Can you work these out from the drawing? Everything is in mm from the part's minimum corner. A direction names the side the tool comes from. Round coordinates to 2 decimals unless told otherwise and drop trailing zeros. Loops run counter-clockwise (first coordinate to the right, second up) from the corner with the lowest first, then second, coordinate; pieces in that order, holes last. Notation, with made-up numbers: M 48,5.25 L 55,5.25 A15 ccw 55,12.25 Z; hole C 0,60.25 d7. An arc over 180 degrees is marked long. Use a Markdown table: item, result.
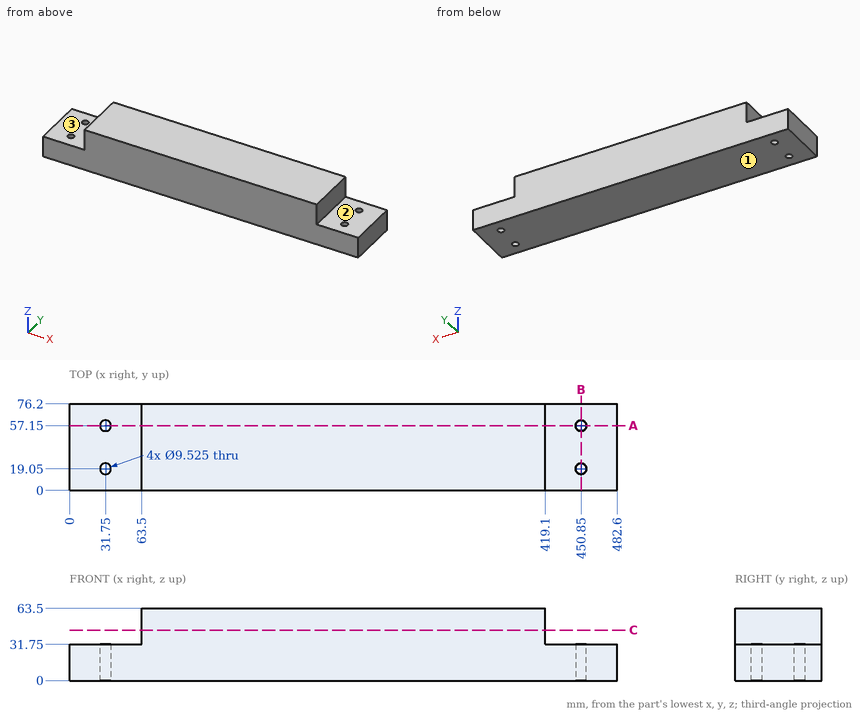
1. Which directions (+Z, -Z, +X, -X, +Y, -Y) give clear straight access to the entire face, cutting with the end or side of a thin tool? Please do the marked faces 1, 2 and 3.
Answer sheet:
| item | result |
|---|---|
| face 1 | -Z, +X, -X, +Y, -Y |
| face 2 | +Z, +X, +Y, -Y |
| face 3 | +Z, -X, +Y, -Y |
2. For pin 1 Ø16 at (y, z) = (40, 50) entering from +X; pin 2 Ø8.5 at (x, y) = (450.85, 57.15) entering from +Z; pin 3 Ø12 at (y, z) = (38.5, 45) entering from -X; pin 4 Ø19 at (x, y) = (20, 39) entering from +Z, each with a flat end and sliding along its axis, tell me the tip position at first contact or that it passes through.
Answer sheet:
| item | result |
|---|---|
| pin 1 | x = 419.1 |
| pin 2 | through |
| pin 3 | x = 63.5 |
| pin 4 | z = 31.75 |
3. Imagine slicing it at C-C, the plane z = 44.5. Write out the boundary of the cut face in (x, y), then the cut area to 3 significant figures.
Answer sheet:
| item | result |
|---|---|
| outline | M 63.5,0 L 419.1,0 L 419.1,76.2 L 63.5,76.2 Z |
| area | 27,100 mm2 |
4. Imagine slicing it at B-B, the plane x = 450.85. Write out the boundary of the cut face in (y, z).
Answer sheet:
| item | result |
|---|---|
| outline | M 0,0 L 14.29,0 L 14.29,31.75 L 0,31.75 Z; M 23.81,0 L 52.39,0 L 52.39,31.75 L 23.81,31.75 Z; M 61.91,0 L 76.2,0 L 76.2,31.75 L 61.91,31.75 Z |
5. I need wall thicknesses on probe 1 along Y at (x, z) = (31.75, 21); probe 2 along X at (y, z) = (19, 23); probe 3 along X at (y, z) = (15, 15). Which ranges of each line are inside material? Lowest first, please. Write a range as from..to.
Answer sheet:
| item | result |
|---|---|
| probe 1 | 0..14.29, 23.81..52.39, 61.91..76.2 |
| probe 2 | 0..26.99, 36.51..446.09, 455.61..482.6 |
| probe 3 | 0..29.24, 34.26..448.34, 453.36..482.6 |
6. Imagine slicing it at A-A, the plane y = 57.15. Write out the boundary of the cut face in (x, z), then the cut area to 3 significant figures.
Answer sheet:
| item | result |
|---|---|
| outline | M 0,0 L 26.99,0 L 26.99,31.75 L 0,31.75 Z; M 36.51,0 L 446.09,0 L 446.09,31.75 L 419.1,31.75 L 419.1,63.5 L 63.5,63.5 L 63.5,31.75 L 36.51,31.75 Z; M 455.61,0 L 482.6,0 L 482.6,31.75 L 455.61,31.75 Z |
| area | 26,000 mm2 |
